Geometry: final body of the model. Coordinates: model frame, mm. A direction names the side the tool comes from. Coordinates: 2 decimals unless noted, no trailing zeros. Loops run counter-clockwise (first coordinate to the right, second up) from the corner with the lowest first, then second, coordinate; pieces in that order, holes last. Notation, with made-up numbers: (32, 73) - (73, 73) arc R9 cw to (73, 88) - close; hole circle Ø7 at (24.5, 27). An arc over 180 degrees is marked (long way). Put each result on its own line as item: value. Start each with the question number.
1) Section C-C on z = -5. Output: boundary loops of the cut face in (x, y), and give its area (3 significant figures).
2) Draft query along Z for faces 1 (the flat face through (0, 17, -8)), 2 (the cylindrical face through (-16.273, 3.951, -0.358)), 3 (the flat face through (-15, 8, 0)), 4 (the flat face through (0, 17, 8)). Return one class per face: +Z half, -Z half, draft (parallel to the pull), parting line (faces both ways), or undercut.
3) Contact query for flat-ended pins moving along their axis: pin 1 Ø3 at (x, z) = (-16.5, -0.5) entering from +Y; pin 2 Ø5 at (x, z) = (8, -1) entering from -Y; pin 3 Ø3 at (y, z) = (30.5, 3.5) entering from -X; pin 4 Ø8 at (y, z) = (27.5, 3.5) entering from +X. Output: stop coordinate, or through.
4) Section B-B on z = 0. Output: boundary loops of the cut face in (x, y), and give its area (3 significant figures).
5) Section A-A on x = 0. Output: boundary loops of the cut face in (y, z), and give its area (3 significant figures).
6) Material intervals for line 1 along X through (y, z) = (6.25, 0); line 2 along X through (y, z) = (35.5, 6.5); line 3 along X through (y, z) = (26, -3.5), sorted ascending. Write a range as from..to.
7) Reachability of faces 5 (the cylindrical face through (-0.976, 34.436, 0.105)), 6 (the flat face through (-12.5, 25, 0)), 7 (the flat face through (16.5, 8, -1.7)) from +Z, -Z, +X, -X, +Y, -Y: full face, straight path, thin tool, end or side. Return the list, or none.
8) Section D-D on x = 19. Output: boundary loops of the cut face in (y, z).
```python
from build123d import *

# Parameters (mm, degrees)
SKETCH_1_W          = 48
SKETCH_1_H          = 16
SKETCH_1_R          = 2.75
EXTRUDE_1_DEPTH     = 8
EXTRUDE_2_DEPTH     = 36
SKETCH_3_R          = 7.5
CUT_EXTRUDE_1_DEPTH = 36
CHAMFER_1_SIZE      = 1
FILLET_1_R          = 0.5


with BuildPart() as part:
    # 草图1 → 凸台-拉伸1 (new body)
    with BuildSketch(Plane(origin=(0, 0, 0), x_dir=(1, 0, 0), z_dir=(0, 1, 0))):
        Rectangle(SKETCH_1_W, SKETCH_1_H)
        with Locations(Location((19, 0, 0), (0, 0, 270))):
            Circle(SKETCH_1_R, mode=Mode.SUBTRACT)
        with Locations(Location((-19, 0, 0), (0, 0, 270))):
            Circle(SKETCH_1_R, mode=Mode.SUBTRACT)
    extrude(amount=EXTRUDE_1_DEPTH)

    # 草图2 → 凸台-拉伸2 (add)
    with BuildSketch(Plane(origin=(0, 8, 0), x_dir=(1, 0, 0), z_dir=(0, 1, 0))):
        Polygon((12.5, -8), (12.5, 8), (-12.5, 8), align=None)
        Polygon((-12.5, -8), (12.5, -8), (-12.5, 8), align=None)
    extrude(amount=EXTRUDE_2_DEPTH)

    # 草图3 → 切除-拉伸1 (cut)
    with BuildSketch(Plane.XY.offset(8)):
        with Locations((0, 27)):
            Circle(SKETCH_3_R)
    extrude(amount=-CUT_EXTRUDE_1_DEPTH, mode=Mode.SUBTRACT)

    # 倒角1
    chamfer_1_edges = [part.edges().sort_by_distance(p)[0] for p in [
        (24, 8, 0),
        (18.25, 8, -8),
        (18.25, 8, 8),
        (-18.25, 8, -8),
        (12.5, 26, -8),
        (-12.5, 26, -8),
        (-12.5, 26, 8),
        (12.5, 44, 0),
        (12.5, 26, 8),
        (0, 44, -8),
        (-12.5, 44, 0),
        (0, 44, 8),
        (-24, 8, 0),
        (0, 0, -8),
        (24, 0, 0),
        (0, 0, 8),
        (-24, 0, 0),
        (-24, 4, -8),
        (24, 4, -8),
        (24, 4, 8),
        (-24, 4, 8),
        (-18.25, 8, 8),
    ]]
    chamfer(chamfer_1_edges, length=CHAMFER_1_SIZE)

    # 圆角1
    fillet_1_edges = [part.edges().sort_by_distance(p)[0] for p in [
        (-19, 0, -2.75),
        (-19, 8, -2.75),
        (-7.5, 27, -8),
        (-7.5, 27, 8),
        (0, 1, 8),
    ]]
    fillet(fillet_1_edges, radius=FILLET_1_R)


solid = part.part
```
Answer block:
1. outline: (-24, 1) - (-23, 0) - (23, 0) - (24, 1) - (24, 7) - (23, 8) - (12.5, 8) - (12.5, 43) - (11.5, 44) - (-11.5, 44) - (-12.5, 43) - (-12.5, 8) - (-23, 8) - (-24, 7) - close; hole circle Ø15 at (0, 27)
1. area: 1,100 mm²
2. face 1: -Z half
2. face 2: undercut
2. face 3: draft
2. face 4: +Z half
3. pin 1: stops at y = 8
3. pin 2: stops at y = 0
3. pin 3: stops at x = -12.5
3. pin 4: stops at x = 12.5
4. outline: (-24, 1) - (-23, 0) - (-22.25, 0) arc R0.5 ccw to (-21.75, 0.5) - (-21.75, 7.5) arc R0.5 ccw to (-22.25, 8) - (-23, 8) - (-24, 7) - close; (-16.25, 0.5) arc R0.5 ccw to (-15.75, 0) - (16.25, 0) - (16.25, 8) - (12.5, 8) - (12.5, 43) - (11.5, 44) - (-11.5, 44) - (-12.5, 43) - (-12.5, 8) - (-15.75, 8) arc R0.5 ccw to (-16.25, 7.5) - close; (21.75, 0) - (23, 0) - (24, 1) - (24, 7) - (23, 8) - (21.75, 8) - close; hole circle Ø15 at (0, 27)
4. area: 1,020 mm²
5. outline: (0, -7) - (1, -8) - (19, -8) arc R0.5 ccw to (19.5, -7.5) - (19.5, 7.5) arc R0.5 ccw to (19, 8) - (1.21, 8) arc R0.5 ccw to (0.85, 7.85) - (0, 7) - close; (34.5, -7.5) arc R0.5 ccw to (35, -8) - (43, -8) - (44, -7) - (44, 7) - (43, 8) - (35, 8) arc R0.5 ccw to (34.5, 7.5) - close
5. area: 462 mm²
6. line 1: x = -24..-21.75, -16.25..16.25, 21.75..24
6. line 2: x = -12.5..12.5
6. line 3: x = -12.5..-7.43, 7.43..12.5
7. face 5: +Z, -Z
7. face 6: +Z, -Z, -X, +Y
7. face 7: +Z, -Z, +X, +Y
8. outline: (0, -7) - (1, -8) - (7, -8) - (8, -7) - (8, -2.75) - (0, -2.75) - close; (0, 2.75) - (8, 2.75) - (8, 7) - (7, 8) - (1.21, 8) arc R0.5 ccw to (0.85, 7.85) - (0, 7) - close
